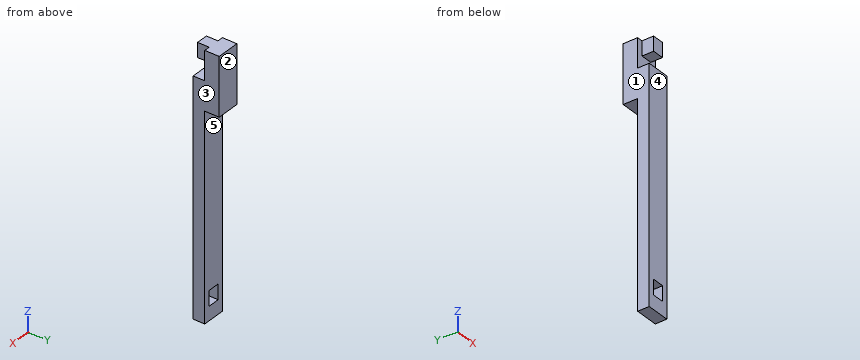
from build123d import *

# Parameters (mm, degrees)
SKETCH_1_W          = 16
SKETCH_1_H          = 160
EXTRUDE_1_DEPTH     = 8
SKETCH_2_W          = 16
SKETCH_2_H          = 20
EXTRUDE_2_DEPTH     = 10
SKETCH_3_W          = 16
SKETCH_3_H          = 10
EXTRUDE_3_DEPTH     = 20
SKETCH_4_W          = 8
SKETCH_4_H          = 10
EXTRUDE_4_DEPTH     = 8
SKETCH_5_W          = 8.4
SKETCH_5_H          = 10.4
CUT_EXTRUDE_1_DEPTH = 162.108658985


with BuildPart() as part:
    # 草图1 → 凸台-拉伸1 (new body)
    with BuildSketch(Plane(origin=(0, 0, 0), x_dir=(1, 0, 0), z_dir=(0, 1, 0))):
        with Locations((8, 80)):
            Rectangle(SKETCH_1_W, SKETCH_1_H)
    extrude(amount=EXTRUDE_1_DEPTH)

    # 草图2 → 凸台-拉伸2 (add)
    with BuildSketch(Plane(origin=(0, 8, 0), x_dir=(1, 0, 0), z_dir=(0, 1, 0))):
        with Locations((8, 10)):
            Rectangle(SKETCH_2_W, SKETCH_2_H)
    extrude(amount=EXTRUDE_2_DEPTH)

    # 草图3 → 凸台-拉伸3 (add)
    with BuildSketch(Plane.XY):
        with Locations((8, 13)):
            Rectangle(SKETCH_3_W, SKETCH_3_H)
    extrude(amount=EXTRUDE_3_DEPTH)

    # 草图4 → 凸台-拉伸4 (add)
    with BuildSketch(Plane.XZ.offset(-8)):
        with Locations((8, 15)):
            Rectangle(SKETCH_4_W, SKETCH_4_H)
    extrude(amount=EXTRUDE_4_DEPTH)

    # 草图5 → 切除-拉伸1 (cut, through all)
    with BuildSketch(Plane(origin=(0, 8, 0), x_dir=(1, 0, 0), z_dir=(0, 1, 0))):
        with Locations((8, 145.2)):
            Rectangle(SKETCH_5_W, SKETCH_5_H)
    extrude(amount=-CUT_EXTRUDE_1_DEPTH, mode=Mode.SUBTRACT)


solid = part.part
The listing builds one solid part. Answer for the finished solid, in the listing's coordinates (mm). Face numbers are marked on the shaded views. A direction names the side the tool comes from. Round coordinates to 2 decimals unless told otherwise and drop trailing zeros. Order: outer loops, then holes, each group sorted by start corner. A loop starts at its lowest first (then second) coordinate and runs counter-clockwise, first axis right, second up. Notation, with made-up numbers: M 87.5,74 L 145.5,74 A27 cw 145.5,99 Z; hole C -15,83 d7. An arc over 180 degrees is marked long. Answer in a Markdown table with one row per item. Add a question column.
1) The part is cut by section C-C on z = -28. Determine the outline of the cut face in (x, y), plus the area to 3 significant figures.
2) The part is cut by section A-A on y = 4. Determine the outline of the cut face in (x, z).
3) Flat-ended cylindrical pins translate along their axes: pin 1 Ø1.5 at (x, y) = (7.5, 11.5) entering from -Z; pin 2 Ø6.5 at (y, z) = (4, 15) entering from -X; pin 3 Ø5 at (x, z) = (11.5, -67) entering from +Y. Find the tip coordinate at first contact, or state that the pin passes through.
4) Which of the six approach directions +Z, -Z, +X, -X, +Y, -Y give full straight-line access (tool end or side, diameter ignored) to the marked faces 4 and 5?
5) The part is cut by section B-B on x = 9.5. Determine the outline of the cut face in (y, z).
6) Determine the mould class of the marked faces 1, 2 and 3 for opening direction X: pulls with the +X half, pulls with the -X half, needs draft (parallel to the pull), parting line crosses it, or undercut.
7) The part is cut by section D-D on y = 15.5. Determine the outline of the cut face in (x, z).
8) Consider line 1 along Z through (x, y) = (6.25, 4.75); line 2 along Z through (x, y) = (10, 14.25); line 3 along Y through (x, z) = (14.75, -30). Determine where each line is inside the solid, lowest interval first. Write a range as from..to.
Findings below:
| question | item | result |
|---|---|---|
| 1 | outline | M 0,0 L 16,0 L 16,8 L 0,8 Z |
| 1 | area | 128 mm² |
| 2 | outline | M 0,-160 L 16,-160 L 16,0 L 0,0 Z; M 4,10 L 12,10 L 12,20 L 4,20 Z; hole M 3.8,-150.4 L 12.2,-150.4 L 12.2,-140 L 3.8,-140 Z |
| 3 | pin 1 | stops at z = -20 |
| 3 | pin 2 | stops at x = 4 |
| 3 | pin 3 | stops at y = 8 |
| 4 | face 4 | +Z, -Z, +X, -X, -Y |
| 4 | face 5 | -Z, +X, -X, +Y |
| 5 | outline | M 0,-160 L 8,-160 L 8,-150.4 L 0,-150.4 Z; M 0,-140 L 8,-140 L 8,-20 L 18,-20 L 18,20 L 0,20 L 0,10 L 8,10 L 8,0 L 0,0 Z |
| 6 | face 1 | pulls with the -X half |
| 6 | face 2 | needs draft |
| 6 | face 3 | pulls with the +X half |
| 7 | outline | M 0,-20 L 16,-20 L 16,20 L 0,20 Z |
| 8 | line 1 | z = -160..-150.4, -140..0, 10..20 |
| 8 | line 2 | z = -20..20 |
| 8 | line 3 | y = 0..8 |
